Geometry check sheet. Reference: the model listing, model coordinates, mm. A direction names the side the tool comes from. Round coordinates to 2 decimals unless told otherwise and drop trailing zeros. Loops run counter-clockwise (first coordinate to the right, second up) from the corner with the lowest first, then second, coordinate; pieces in that order, holes last. Notation, with made-up numbers: (-32.5, 53) - (-5.5, 53) arc R24 ccw to (-5.5, 65) - close; hole circle Ø6 at (49, 57). An arc over 180 degrees is marked (long way). Write item = value, one per line.
```python
from build123d import *

# Parameters (mm, degrees)
CUT_EXTRUDE2_OUTLINE_R   = 2.5019
CUT_EXTRUDE2_DEPTH       = 5.4864
CUT_EXTRUDE2_START       = -238.9886
CUT_EXTRUDE2_2_DEPTH     = 238.9886
CUT_EXTRUDE2_START_2     = -1
CUT_EXTRUDE2_3_DEPTH     = 124
CUT_EXTRUDE2_START_3     = 120.015
CUT_EXTRUDE2_4_OUTLINE_R = 1.7526
CUT_EXTRUDE2_4_DEPTH     = 2.985
CHAMFER1_SIZE            = 0.635
CHAMFER2_SIZE            = 0.635
CUT_EXTRUDE3_START       = -0.9906
SKETCH2_R                = 1.7526
CUT_EXTRUDE3_DEPTH       = 0.9906
CHAMFER3_SIZE            = 0.635


with BuildPart() as part:
    # Cut-Extrude2: read off the stored shape, not the designer's step
    # Cut-Extrude2 outline → Cut-Extrude2 (new body)
    with BuildSketch(Plane(origin=(0, 0, 0), x_dir=(1, 0, 0), z_dir=(0, 1, 0))):
        with Locations((113.6904, 201.6252)):
            Circle(CUT_EXTRUDE2_OUTLINE_R)
        with Locations((80.4418, 93.3704)):
            Circle(CUT_EXTRUDE2_OUTLINE_R)
        with Locations((113.6904, 5.9944)):
            Circle(CUT_EXTRUDE2_OUTLINE_R)
        with Locations((8.6868, 5.9944)):
            Circle(CUT_EXTRUDE2_OUTLINE_R)
        with Locations((8.6868, 226.9998)):
            Circle(CUT_EXTRUDE2_OUTLINE_R)
    extrude(amount=CUT_EXTRUDE2_DEPTH)

    # Cut-Extrude2 2 outline → Cut-Extrude2 2 (add)
    with BuildSketch(Plane.XY.offset(CUT_EXTRUDE2_START)):
        with BuildLine():
            Line((121.9962, 1.9812), (121.9962, 43.0022))
            Line((121.9962, 43.0022), (121.0056, 43.0022))
            Line((121.0056, 43.0022), (121.0056, 1.9812))
            ThreePointArc((121.0056, 1.9812), (120.715459977, 1.280740023), (120.015, 0.9906))
            Line((120.015, 0.9906), (1.9812, 0.9906))
            ThreePointArc((1.9812, 0.9906), (1.280740019, 1.280740026), (0.9906, 1.98120001))
            Line((0.9906, 1.98120001), (0.9906, 43.0022))
            Line((0.9906, 43.0022), (0, 43.0022))
            Line((0, 43.0022), (0, 1.98120001))
            ThreePointArc((0, 1.98120001), (0.580280042, 0.580280049), (1.9812, 0))
            Line((1.9812, 0), (120.014999999, 0))
            ThreePointArc((120.014999999, 0), (121.415919955, 0.580280045), (121.9962, 1.9812))
        make_face()
    extrude(amount=CUT_EXTRUDE2_2_DEPTH)

    # Cut-Extrude2 3 outline → Cut-Extrude2 3 (cut)
    with BuildSketch(Plane.YZ.offset(CUT_EXTRUDE2_START_2)):
        Polygon((43.0022, 0), (0.9906, 0), (43.002200003, -14.706600001), align=None)
    extrude(amount=CUT_EXTRUDE2_3_DEPTH, mode=Mode.SUBTRACT)

    # Cut-Extrude2 4 outline → Cut-Extrude2 4 (cut)
    with BuildSketch(Plane.YZ.offset(CUT_EXTRUDE2_START_3)):
        with Locations((37.0078, -23.1902)):
            Circle(CUT_EXTRUDE2_4_OUTLINE_R)
        with Locations((37.0078, -174.5996)):
            Circle(CUT_EXTRUDE2_4_OUTLINE_R)
    extrude(amount=CUT_EXTRUDE2_4_DEPTH, mode=Mode.SUBTRACT)

    # Chamfer1
    chamfer1_edges = [part.edges().sort_by_distance(p)[0] for p in [
        (121.9962, 35.2552, -23.1902),
    ]]
    chamfer(chamfer1_edges, length=CHAMFER1_SIZE)

    # Chamfer2
    chamfer2_edges = [part.edges().sort_by_distance(p)[0] for p in [
        (121.9962, 35.2552, -174.5996),
    ]]
    chamfer(chamfer2_edges, length=CHAMFER2_SIZE)

    # Sketch2 → Cut-Extrude3 (cut)
    with BuildSketch(Plane(origin=(0.9906, 0, 0), x_dir=(0, 0, -1), z_dir=(1, 0, 0)).offset(CUT_EXTRUDE3_START)):
        with Locations(Location((23.1902, 37.0078, 0), (0, 0, 180))):
            Circle(SKETCH2_R)
        with Locations(Location((174.5996, 37.0078, 0), (0, 0, 180))):
            Circle(SKETCH2_R)
    extrude(amount=CUT_EXTRUDE3_DEPTH, mode=Mode.SUBTRACT)

    # Chamfer3
    chamfer3_edges = [part.edges().sort_by_distance(p)[0] for p in [
        (0, 37.0078, -24.9428),
        (0, 37.0078, -176.3522),
    ]]
    chamfer(chamfer3_edges, length=CHAMFER3_SIZE)


solid = part.part
```
(1) Scan lines: L1, parallel to X at y = 23.5, z = -110.5; L2, parallel to Y at x = 99.5, z = -178. Record each from-to range of solid material in increasing order. Write a range as [from, to].
Answers follow:
L1 = [0, 0.99], [121.01, 122]
L2 = [0, 0.99]
(2) Gauge pin test, flat ends, axial feed: pin 1 (4 mm diameter, centred on x = 113, z = -200.5, fed in from +Y); pin 2 (3 mm diameter, centred on y = 37.01, z = -174.6, fed in from +X). Record the tip position at first contact, or that the pin passes through.
Answers follow:
pin_1 = 5.49
pin_2 = through
(3) Mould release check, pull along X, two halves, no side actions. Record for faces 1 (the flat face through (0, 23, -121)), 2 (the flat face through (121.996, 22, -121)), 3 (the flat face through (80, 5.486, -93)), 4 (the flat face through (121.43, 21.7, -7.25)): pulls with the +X half, pulls with the -X half, needs draft (parallel to the pull), parting line crosses it, or undercut.
Answers follow:
face_1 = pulls with the -X half
face_2 = pulls with the +X half
face_3 = undercut
face_4 = needs draft
(4) Section check B-B (z = -17). Enter the section's corners in (x, y) (3 decimals), then the cut area to 3 significant figures.
Answers follow:
outline = (0, 1.981) arc R1.981 ccw to (1.981, 0) - (120.015, 0) arc R1.981 ccw to (121.996, 1.981) - (121.996, 43.002) - (121.006, 43.002) - (121.006, 1.981) arc R0.991 cw to (120.015, 0.991) - (1.981, 0.991) arc R0.991 cw to (0.991, 1.981) - (0.991, 43.002) - (0, 43.002) - close
area = 203 mm²
(5) Section check A-A (y = 21). Enter the section's corners in (x, z).
Answers follow:
outline = (0, -238.99) - (0.99, -238.99) - (0.99, -7) - (0, -7) - close; (121.01, -238.99) - (122, -238.99) - (122, -7) - (121.01, -7) - close
(6) Set-up check for faces 5 (the flat face through (114, 5.486, -202)), 6 (the flat face through (0.54, 21.7, -7.25)), 7 (the cylindrical face through (6.843, 3.207, -7.685)): record each of +Z, -Z, +X, -X, +Y, -Y from which the full face is reachable in a straight line by a thin tool's end or side.
Answers follow:
face_5 = +Z, -Z, +Y
face_6 = +Z, +X, -X, +Y
face_7 = +Y
(7) Section check C-C (x = 54). Enter the section's corners in (y, z).
Answers follow:
outline = (0, -238.99) - (0.99, -238.99) - (0.99, 0) - (0, 0) - close
